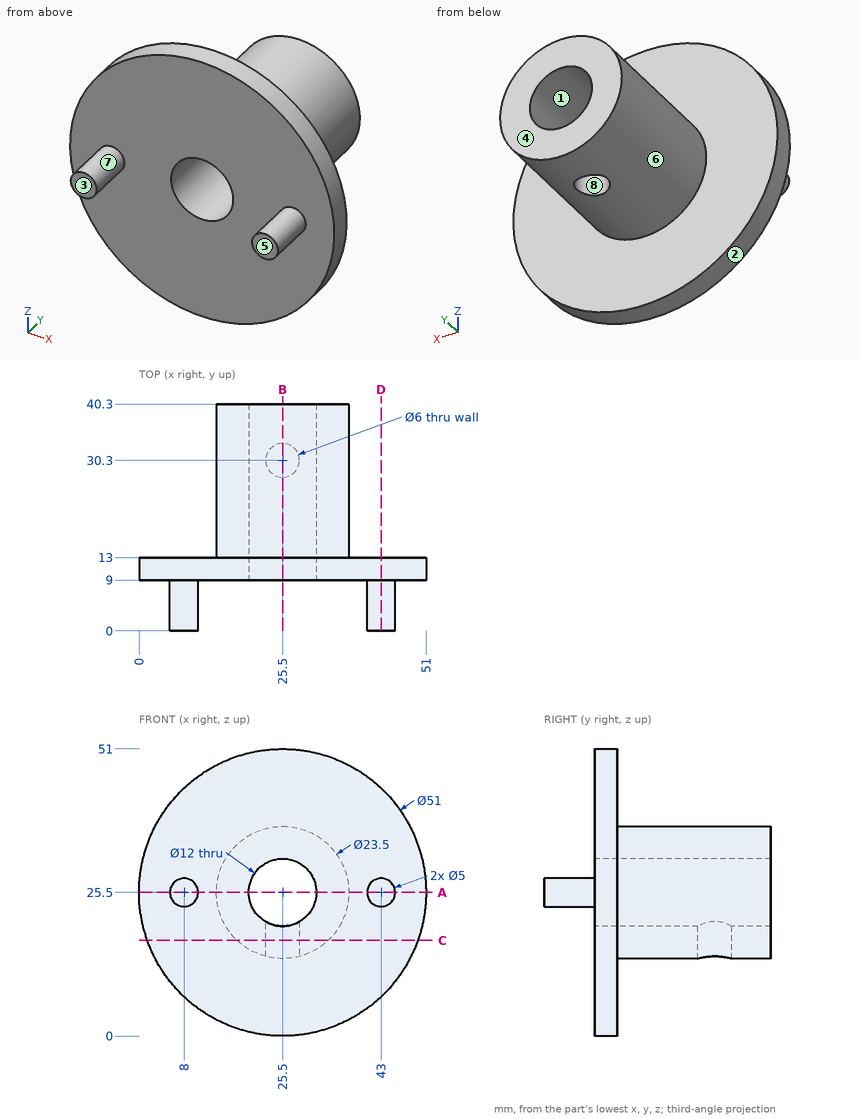
The figure shows three views and two pictorial views of one solid part (mm, origin at its lowest corner). Answer the questions. A direction names the side the tool comes from. Give positions to 0.01 mm unless a question says otherwise; leave off trailing zeros. Write each loop counter-clockwise with the first axis right and the second up, starting at its lowest first coordinate (ties: lowest second). Pieces come first, ordered by that corner, then holes. Notation, with made-up numbers: (35, -10.75) - (55, -10.75) arc R16 cw to (55, -6.75) - close; hole circle Ø8 at (54, -2.5). An arc over 180 degrees is marked (long way). Use CSV: the item, a comma, the result in double quotes. Start each with the question number.
Item 1: Flat-ended cylindrical pins translate along their axes: P1, Ø1.5, axis at y = 11, z = 17.5, coming from the +X side; P2, Ø3, axis at x = 39.5, y = 5.5, coming from the +Z side; P3, Ø2, axis at y = 15.5, z = 24, coming from the -X side. Find the tip coordinate at first contact, or state that the pin passes through.
Item 2: The part is cut by section B-B, the plane x = 25.5. Give the vertices of the cut face in (y, z), and give its area (3 significant figures).
Item 3: Consider line 1 (X direction, y = 16, z = 25.5); line 2 (Y direction, x = 23, z = 48.5); line 3 (X direction, y = 30, z = 18). Determine where each line is inside the solid, lowest interval first.
Item 4: The part is cut by section A-A, the plane z = 25.5. Give the vertices of the cut face in (x, y), and give its area (3 significant figures).
Item 5: For the marked faces 4, 5, 6, 7 and 8, determine the directions among +Z, -Z, +X, -X, +Y, -Y from which every point of the face is accessible in a straight line to the end or side of a thin tool.
Item 6: The part is cut by section C-C, the plane z = 17. Give the vertices of the cut face in (x, y).
Item 7: The mould has two halves that part along X. Classify the marked faces 1, 2 and 3: pulls with the +X half, pulls with the -X half, needs draft (parallel to the pull), parting line crosses it, or undercut.
Item 8: The part is cut by section D-D, the plane x = 43. Give the vertices of the cut face in (y, z).
Taken from the geometry:
1,P1,"x = 49.95"
1,P2,"z = 27"
1,P3,"x = 13.76"
2,outline,"(9, 0) - (13, 0) - (13, 13.75) - (27.3, 13.75) - (27.3, 19.5) - (9, 19.5) - close; (9, 31.5) - (40.3, 31.5) - (40.3, 37.25) - (13, 37.25) - (13, 51) - (9, 51) - close; (33.3, 13.75) - (40.3, 13.75) - (40.3, 19.5) - (33.3, 19.5) - close"
2,area,"435 mm2"
3,line 1,"13.75 to 19.5, 31.5 to 37.25"
3,line 2,"9 to 13"
3,line 3,"16.45 to 22.52, 28.48 to 34.55"
4,outline,"(0, 9) - (5.5, 9) - (5.5, 0) - (10.5, 0) - (10.5, 9) - (19.5, 9) - (19.5, 40.3) - (13.75, 40.3) - (13.75, 13) - (0, 13) - close; (31.5, 9) - (40.5, 9) - (40.5, 0) - (45.5, 0) - (45.5, 9) - (51, 9) - (51, 13) - (37.25, 13) - (37.25, 40.3) - (31.5, 40.3) - close"
4,area,"560 mm2"
5,face 4,"+Z, -Z, +X, -X, +Y"
5,face 5,"+Z, -Z, +X, -X, -Y"
5,face 6,"+Y"
5,face 7,"-Y"
5,face 8,"-Z"
6,outline,"(1.46, 9) - (49.54, 9) - (49.54, 13) - (33.61, 13) - (33.61, 40.3) - (17.39, 40.3) - (17.39, 13) - (1.46, 13) - close; hole circle Ø6 at (25.5, 30.3)"
7,face 1,"undercut"
7,face 2,"parting line crosses it"
7,face 3,"needs draft"
8,outline,"(0, 23) - (9, 23) - (9, 6.95) - (13, 6.95) - (13, 44.05) - (9, 44.05) - (9, 28) - (0, 28) - close"
